```python
from build123d import *

# Parameters (mm, degrees)
EXTRUDE_1_DEPTH    = 8
HOLE_WIZARD_M6_1_D = 5
HOLE_WIZARD_M6_2_D = 5
HOLE_WIZARD_M6_3_D = 5


with BuildPart() as part:
    # 草图1 → 凸台-拉伸1 (new body)
    with BuildSketch(Plane.XY):
        Polygon((0, 0), (28, 0), (28, 6.360297657), (18, 10), (10, 10), (0, 6.360297657), align=None)
    extrude(amount=-EXTRUDE_1_DEPTH)

    # M6 螺纹孔1 (through all)
    with Locations(Plane(origin=(0, 10, 0), x_dir=(1, 0, 0), z_dir=(0, 1, 0))):
        with Locations((14, 4)):
            Hole(HOLE_WIZARD_M6_1_D / 2)

    # M6 螺纹孔2 (through all)
    with Locations(Plane(origin=(5.31953806, 14.615310703, 0), x_dir=(0.9396926207859093, -0.34202014332566627, 0), z_dir=(0.34202014332566627, 0.9396926207859093, 0))):
        with Locations((20.636043466, 4)):
            Hole(HOLE_WIZARD_M6_2_D / 2)

    # M6 螺纹孔3 (through all)
    with Locations(Plane(origin=(-2.044160264, 5.616284167, 0), x_dir=(0.9396926207859093, 0.3420201433256663, 0), z_dir=(-0.3420201433256663, 0.9396926207859093, 0))):
        with Locations((5.675349916, 4)):
            Hole(HOLE_WIZARD_M6_3_D / 2)


solid = part.part
```
Check sheet for the modelled part. Datum: model origin and axes. Units: mm. Round coordinates to 2 decimals unless told otherwise and drop trailing zeros. Write each loop counter-clockwise with the first axis right and the second up, starting at its lowest first coordinate (ties: lowest second). Pieces come first, ordered by that corner, then holes. Notation, with made-up numbers: (20, 59.25) -> (30, 59.25) arc R15 cw to (30, 68.25) -> close; hole circle Ø2 at (70.5, -0.5). An arc over 180 degrees is marked (long way). Put each result on its own line as item: value.
(1) Material ranges on line 1 (Z direction, x = 14, y = 7.75); line 2 (X direction, y = 1.5, z = -6.25); line 3 (Z direction, x = 16.25, y = 6.5), recorded low to high.
Values found:
line 1: z = -8 to -6.5, -1.5 to 0
line 2: x = 0 to 4.33, 6.65 to 12.91, 15.09 to 21.35, 23.67 to 28
line 3: z = -8 to -5.09, -2.91 to 0
(2) Sectioned sample at D-D (z = -4). Enter the section's corners in (x, y), plus the area to 3 significant figures.
Values found:
outline: (0, 0) -> (3.38, 0) -> (0.94, 6.7) -> (0, 6.36) -> close; (5.64, 8.41) -> (8.7, 0) -> (11.5, 0) -> (11.5, 10) -> (10, 10) -> close; (16.5, 0) -> (19.3, 0) -> (22.36, 8.41) -> (18, 10) -> (16.5, 10) -> close; (24.62, 0) -> (28, 0) -> (28, 6.36) -> (27.06, 6.7) -> close
area: 113 mm^2
(3) Mould release check, pull along Z, two halves, no side actions. Record for faces 1 (the face through (21.96, 8.56, -3.94)), 2 (the face through (15.84, 4.93, -5.69)), 3 (the face through (14, 4, -8)): released by +Z, released by -Z, zero draft, split by the parting line, or undercut.
Values found:
face 1: zero draft
face 2: undercut
face 3: released by -Z
(4) Sectioned sample at C-C (y = 5.5). Count the separate pieces of the cut face and the enclosed holes in it, plus the area to 3 significant figures.
Values found:
separate pieces: 1
enclosed holes: 3
area: 163 mm^2
(5) Sectioned sample at B-B (z = -5.5). Enter the section's corners in (x, y).
Values found:
outline: (0, 0) -> (3.91, 0) -> (1.41, 6.87) -> (0, 6.36) -> close; (5.17, 8.24) -> (8.17, 0) -> (12, 0) -> (12, 10) -> (10, 10) -> close; (16, 0) -> (19.83, 0) -> (22.83, 8.24) -> (18, 10) -> (16, 10) -> close; (24.09, 0) -> (28, 0) -> (28, 6.36) -> (26.59, 6.87) -> close
(6) Sectioned sample at A-A (x = 14). Enter the section's corners in (y, z), plus the area to 3 significant figures.
Values found:
outline: (0, -8) -> (10, -8) -> (10, -6.5) -> (0, -6.5) -> close; (0, -1.5) -> (10, -1.5) -> (10, 0) -> (0, 0) -> close
area: 30.0 mm^2
